from build123d import *

# Parameters (mm, degrees)
SKETCH1_R           = 85
BOSS_EXTRUDE1_DEPTH = 4
SKETCH2_R           = 4.25
CUT_EXTRUDE1_DEPTH  = 5
CUT_EXTRUDE2_DEPTH  = 5
SKETCH5_W           = 42.180521306
SKETCH5_H           = 70
CUT_EXTRUDE4_DEPTH  = 5
SKETCH6_W           = 106.727452964
SKETCH6_H           = 15
BOSS_EXTRUDE3_DEPTH = 4
SKETCH7_R           = 70
CUT_EXTRUDE5_DEPTH  = 5
SKETCH8_R           = 2.25
CUT_EXTRUDE6_DEPTH  = 5
LPATTERN1_COUNT     = 3
LPATTERN1_PITCH     = 10
FILLET1_R           = 10
FILLET2_R           = 2


with BuildPart() as part:
    # Sketch1 → Boss-Extrude1 (new body)
    with BuildSketch(Plane(origin=(0, 0, 0), x_dir=(1, 0, 0), z_dir=(0, 1, 0))):
        Circle(SKETCH1_R)
    extrude(amount=BOSS_EXTRUDE1_DEPTH)

    # Sketch2 → Cut-Extrude1 (cut, through all)
    with BuildSketch(Plane(origin=(0, 4, 0), x_dir=(1, 0, 0), z_dir=(0, 1, 0))):
        with Locations((-54.800775542, 54.800775542)):
            Circle(SKETCH2_R)
    extrude(amount=-CUT_EXTRUDE1_DEPTH, mode=Mode.SUBTRACT)

    # Sketch3 → Cut-Extrude2 (cut, through all)
    with BuildSketch(Plane(origin=(0, 4, 0), x_dir=(1, 0, 0), z_dir=(0, 1, 0))):
        with BuildLine():
            Line((0, 0), (-85, 0))
            ThreePointArc((-85, 0), (76.71974917, -36.593443229), (-53.492233239, 66.057406724))
            Line((-53.492233239, 66.057406724), (0, 0))
        make_face()
    extrude(amount=-CUT_EXTRUDE2_DEPTH, mode=Mode.SUBTRACT)

    # Sketch5 → Cut-Extrude4 (cut, through all)
    with BuildSketch(Plane(origin=(0, 0, 0), x_dir=(1, 0, 0), z_dir=(0, 1, 0))):
        with Locations((-74.50134639, 0)):
            Rectangle(SKETCH5_W, SKETCH5_H)
    extrude(amount=CUT_EXTRUDE4_DEPTH, mode=Mode.SUBTRACT)

    # Sketch6 → Boss-Extrude3 (add)
    with BuildSketch(Plane(origin=(0, 0, 0), x_dir=(1, 0, 0), z_dir=(0, 1, 0))):
        with Locations((-94.095940442, 35)):
            Rectangle(SKETCH6_W, SKETCH6_H)
    extrude(amount=BOSS_EXTRUDE3_DEPTH)

    # Sketch7 → Cut-Extrude5 (cut, through all)
    with BuildSketch(Plane(origin=(0, 0, 0), x_dir=(1, 0, 0), z_dir=(0, 1, 0))):
        Circle(SKETCH7_R)
    extrude(amount=CUT_EXTRUDE5_DEPTH, mode=Mode.SUBTRACT)

    # Sketch8 → Cut-Extrude6 (cut, through all)
    with BuildSketch(Plane(origin=(0, 4, 0), x_dir=(1, 0, 0), z_dir=(0, 1, 0))):
        with Locations((-139.959666924, 35)):
            Circle(SKETCH8_R)
    cut_extrude6 = extrude(amount=-CUT_EXTRUDE6_DEPTH, mode=Mode.SUBTRACT)

    # LPattern1: Cut-Extrude6 ×3
    with Locations(*[(i * LPATTERN1_PITCH, 0, 0) for i in range(1, LPATTERN1_COUNT)]):
        add(cut_extrude6, mode=Mode.SUBTRACT)

    # Fillet1
    fillet1_edges = [part.edges().sort_by_distance(p)[0] for p in [
        (-73.612159322, 2, -42.5),
        (-64.371965948, 2, -27.5),
    ]]
    fillet(fillet1_edges, radius=FILLET1_R)

    # Fillet2
    fillet2_edges = [part.edges().sort_by_distance(p)[0] for p in [
        (-53.492233239, 2, -66.057406724),
        (-44.052427373, 2, -54.400217302),
    ]]
    fillet(fillet2_edges, radius=FILLET2_R)


solid = part.part
Here's how the part is built. I have some questions about the finished solid (model axes, mm). Round coordinates to 2 decimals unless told otherwise and drop trailing zeros. Order: outer loops, then holes, each group sorted by start corner. A loop starts at its lowest first (then second) coordinate and runs counter-clockwise, first axis right, second up. Notation, with made-up numbers: (-1.5, -34.75) -> (19.5, -34.75) arc R5 cw to (19.5, -28.75) -> close; hole circle Ø3 at (-14.75, 56.25). An arc over 180 degrees is marked (long way). Return JSON: item names as keys, results as strings.
Q1. For pin 1 Ø1.2 at (x, y) = (-106, 2.5) entering from -Z; pin 2 Ø8 at (x, z) = (-85.5, -44) entering from -Y, each with a flat end and sliding along its axis, tell me the tip position at first contact or that it passes through.
Filled sheet:
{"pin 1": "stops at z = -42.5", "pin 2": "stops at y = 0"}
Q2. I need wall thicknesses on line 1 along X through (y, z) = (3.8, -54.5); line 2 along X through (y, z) = (3.45, -37); line 3 along X through (y, z) = (1.35, -35). Which ranges of each line are inside material? Lowest first, please. Write a range as from..to.
Filled sheet:
{"line 1": "x = -65.23..-59.04, -50.56..-44.86", "line 2": "x = -147.46..-140.99, -138.93..-130.99, -128.93..-120.99, -118.93..-59.42", "line 3": "x = -147.46..-142.21, -137.71..-132.21, -127.71..-122.21, -117.71..-60.62"}
Q3. If we section it at B-B on z = -35: List the corners of the cut face in (x, y) for me, plus the area to 3 significant figures.
Filled sheet:
{"outline": "(-147.46, 0) -> (-142.21, 0) -> (-142.21, 4) -> (-147.46, 4) -> close; (-137.71, 0) -> (-132.21, 0) -> (-132.21, 4) -> (-137.71, 4) -> close; (-127.71, 0) -> (-122.21, 0) -> (-122.21, 4) -> (-127.71, 4) -> close; (-117.71, 0) -> (-60.62, 0) -> (-60.62, 4) -> (-117.71, 4) -> close", "area": "293 mm^2"}
Q4. If we section it at C-C on y = 3.1: List the corners of the cut face in (x, z) for me, plus the area to 3 significant figures.
Filled sheet:
{"outline": "(-147.46, -42.5) -> (-79.18, -42.5) arc R10 cw to (-70.84, -46.97) arc R85 ccw to (-55.07, -64.75) arc R2 ccw to (-52.22, -64.48) -> (-45.29, -55.93) arc R2 ccw to (-45.55, -53.16) arc R70 cw to (-61.83, -32.81) arc R10 ccw to (-70.67, -27.5) -> (-147.46, -27.5) -> close; hole circle Ø4.5 at (-139.96, -35); hole circle Ø4.5 at (-129.96, -35); hole circle Ø4.5 at (-119.96, -35); hole circle Ø8.5 at (-54.8, -54.8)", "area": "1,560 mm^2"}
Q5. If we section it at D-D on x = -94: List the corners of the cut face in (y, z) for me, plus the area to 3 significant figures.
Filled sheet:
{"outline": "(0, -42.5) -> (4, -42.5) -> (4, -27.5) -> (0, -27.5) -> close", "area": "60.0 mm^2"}
Q6. If we section it at A-A on x = -130: List the corners of the cut face in (y, z) for me, plus the area to 3 significant figures.
Filled sheet:
{"outline": "(0, -42.5) -> (4, -42.5) -> (4, -37.25) -> (0, -37.25) -> close; (0, -32.75) -> (4, -32.75) -> (4, -27.5) -> (0, -27.5) -> close", "area": "42.0 mm^2"}
Q7. If we mould it in two halves opening along Z, with no side actions, what happens to faces 1 (the flat face through (-110, 2, -27.5)), 2 (the flat face through (-114, 2, -42.5)), 3 (the cylindrical face through (-137.814, 2.028, -35.676))? For each: released by +Z, released by -Z, zero draft, split by the parting line, or undercut.
Filled sheet:
{"face 1": "released by +Z", "face 2": "released by -Z", "face 3": "undercut"}
